from build123d import *

# Parameters (mm, degrees)
SKETCH1_W           = 130
SKETCH1_H           = 35
BOSS_EXTRUDE1_DEPTH = 6.35
SKETCH5_R           = 3.18
CUT_EXTRUDE2_DEPTH  = 135.778790987
SKETCH8_R           = 2.58660254
CUT_EXTRUDE4_DEPTH  = 135.778790987


with BuildPart() as part:
    # Sketch1 → Boss-Extrude1 (new body)
    with BuildSketch(Plane(origin=(0, 0, 0), x_dir=(1, 0, 0), z_dir=(0, 1, 0))):
        with Locations((65, -17.5)):
            Rectangle(SKETCH1_W, SKETCH1_H)
    extrude(amount=BOSS_EXTRUDE1_DEPTH)

    # Sketch5 → Cut-Extrude2 (cut, through all)
    with BuildSketch(Plane(origin=(0, 6.35, 0), x_dir=(1, 0, 0), z_dir=(0, 1, 0))):
        with Locations(Location((8.605, -17.382603272, 0), (0, 0, 270))):
            Circle(SKETCH5_R)
        with Locations(Location((121.395, -17.382603272, 0), (0, 0, 270))):
            Circle(SKETCH5_R)
    extrude(amount=-CUT_EXTRUDE2_DEPTH, mode=Mode.SUBTRACT)

    # Sketch8 → Cut-Extrude4 (cut, through all)
    with BuildSketch(Plane.XZ):
        with Locations(Location((30.060178317, 15.396500763, 0), (0, 0, 270))):
            Circle(SKETCH8_R)
        with Locations((30.060178317, 36.396500763)):
            Circle(SKETCH8_R)
        with Locations((58.060178317, 36.396500763)):
            Circle(SKETCH8_R)
        with Locations(Location((58.060178317, 15.396500763, 0), (0, 0, 270))):
            Circle(SKETCH8_R)
        with Locations(Location((75.642130445, 15.396500763, 0), (0, 0, 270))):
            Circle(SKETCH8_R)
        with Locations((75.642130445, 36.396500763)):
            Circle(SKETCH8_R)
        with Locations(Location((103.642130445, 15.396500763, 0), (0, 0, 270))):
            Circle(SKETCH8_R)
        with Locations((103.642130445, 36.396500763)):
            Circle(SKETCH8_R)
    extrude(amount=-CUT_EXTRUDE4_DEPTH, mode=Mode.SUBTRACT)


solid = part.part
Design review of the part built by this model. Coordinates are the model's own, in mm. Round coordinates to 2 decimals unless told otherwise and drop trailing zeros. Write each loop counter-clockwise with the first axis right and the second up, starting at its lowest first coordinate (ties: lowest second). Pieces come first, ordered by that corner, then holes. Notation, with made-up numbers: (73, 36) - (88, 36) arc R20 cw to (88, 68) - close; hole circle Ø4 at (-21, 38.25). An arc over 180 degrees is marked (long way). Use a Markdown table: item, result. Add a question column.
1. We need section C-C (z = 16). State the section outline as (x, y) points.
2. We need section B-B (y = 2.25). State the section outline as (x, z) points (1 decimal).
3. Clearance check with a flat-ended pin moving along its axis: pin 1 (5.5 mm diameter, centred on x = 8.6, z = 17.38, fed in from +Y). State where the tip first meets the part, or that it passes through.
4. Mouldability with a two-part tool opening along X and no side actions: class faces 1 (the face through (14, 3, 35)), 2 (the face through (75.61, 3.13, 33.81)), 3 (the face through (130, 3, 18)) as +X half, -X half, draft (parallel to the pull), parting line (faces both ways), or undercut.
5. We need section A-A (x = 119.5). State the section outline as (y, z) points, then the cut area to 3 significant figures.
6. Wall thickness on probe 1 along X at (y, z) = (3.75, 14); probe 2 along Z at (x, y) = (103.5, 5.75); probe 3 along Z at (x, y) = (121.5, 0.5): over which ranges is each line inside the solid? List them lowest first.
Output:
| question | item | result |
|---|---|---|
| 1 | outline | (0, 0) - (5.74, 0) - (5.74, 6.35) - (0, 6.35) - close; (11.47, 0) - (27.54, 0) - (27.54, 6.35) - (11.47, 6.35) - close; (32.58, 0) - (55.54, 0) - (55.54, 6.35) - (32.58, 6.35) - close; (60.58, 0) - (73.13, 0) - (73.13, 6.35) - (60.58, 6.35) - close; (78.16, 0) - (101.13, 0) - (101.13, 6.35) - (78.16, 6.35) - close; (106.16, 0) - (118.53, 0) - (118.53, 6.35) - (106.16, 6.35) - close; (124.26, 0) - (130, 0) - (130, 6.35) - (124.26, 6.35) - close |
| 2 | outline | (0, 0) - (130, 0) - (130, 35) - (105.8, 35) arc R2.6 cw to (101.5, 35) - (77.8, 35) arc R2.6 cw to (73.5, 35) - (60.2, 35) arc R2.6 cw to (55.9, 35) - (32.2, 35) arc R2.6 cw to (27.9, 35) - (0, 35) - close; hole circle Ø6.4 at (8.6, 17.4); hole circle Ø5.2 at (30.1, 15.4); hole circle Ø5.2 at (58.1, 15.4); hole circle Ø5.2 at (75.6, 15.4); hole circle Ø5.2 at (103.6, 15.4); hole circle Ø6.4 at (121.4, 17.4) |
| 3 | pin 1 | passes through |
| 4 | face 1 | draft |
| 4 | face 2 | undercut |
| 4 | face 3 | +X half |
| 5 | outline | (0, 0) - (6.35, 0) - (6.35, 14.83) - (0, 14.83) - close; (0, 19.94) - (6.35, 19.94) - (6.35, 35) - (0, 35) - close |
| 5 | area | 190 mm2 |
| 6 | probe 1 | x = 0 to 27.88, 32.24 to 55.88, 60.24 to 73.46, 77.82 to 101.46, 105.82 to 130 |
| 6 | probe 2 | z = 0 to 12.81, 17.98 to 33.81 |
| 6 | probe 3 | z = 0 to 14.2, 20.56 to 35 |
